```python
from build123d import *

# Parameters (mm, degrees)
EXTRUDE_1_DEPTH = 1
SKETCH_3_R      = 1.5
SKETCH_3_R_2    = 2.75
EXTRUDE_2_DEPTH = 6
EXTRUDE_3_DEPTH = 3


with BuildPart() as part:
    # 草图1 → 凸台-拉伸1 (new body)
    with BuildSketch(Plane.XY):
        with BuildLine():
            Line((-15.782608696, 8.75), (17.217391304, 8.75))
            ThreePointArc((17.217391304, 8.75), (20.045818429, 7.578427125), (21.217391304, 4.75))
            Line((21.217391304, 4.75), (21.217391304, -3.25))
            ThreePointArc((21.217391304, -3.25), (20.045818429, -6.078427125), (17.217391304, -7.25))
            Line((17.217391304, -7.25), (-15.782608696, -7.25))
            ThreePointArc((-15.782608696, -7.25), (-18.61103582, -6.078427125), (-19.782608696, -3.25))
            Line((-19.782608696, -3.25), (-19.782608696, 4.75))
            ThreePointArc((-19.782608696, 4.75), (-18.61103582, 7.578427125), (-15.782608696, 8.75))
        make_face()
    extrude(amount=EXTRUDE_1_DEPTH)

    # 草图3 → 凸台-拉伸2 (add)
    with BuildSketch(Plane.XY.offset(1)):
        with Locations((2.717391304, 5.25)):
            Circle(SKETCH_3_R)
        with Locations((9.717391304, 5.25)):
            Circle(SKETCH_3_R)
        with Locations((6.217391304, -2.75)):
            Circle(SKETCH_3_R_2)
        with Locations((15.717391304, -0.75)):
            Circle(SKETCH_3_R_2)
    extrude(amount=EXTRUDE_2_DEPTH)

    # 草图4 → 凸台-拉伸3 (add)
    with BuildSketch(Plane.XY):
        Polygon((-8.282608696, 2.75), (-8.282608696, 6.75), (-12.282608696, 6.75), (-12.282608696, 2.75), (-16.282608696, 2.75), (-16.282608696, -1.25), (-12.282608696, -1.25), (-12.282608696, -5.25), (-8.282608696, -5.25), (-8.282608696, -1.25), (-4.282608696, -1.25), (-4.282608696, 2.75), align=None)
    extrude(amount=EXTRUDE_3_DEPTH)


solid = part.part
```
Here's how the part is built. I have some questions about the finished solid (model axes, mm). A direction names the side the tool comes from. Give positions to 0.01 mm unless a question says otherwise; leave off trailing zeros. Loops run counter-clockwise (first coordinate to the right, second up) from the corner with the lowest first, then second, coordinate; pieces in that order, holes last. Notation, with made-up numbers: M 13,86 L 21,86 A19 cw 21,93 Z; hole C 75.25,45 d9. An arc over 180 degrees is marked long. Use one line per item in the form item = value. Start each with the question number.
Q1. Thinking about a two-plate mould opening in X: for faces 5 (the cylindrical face through (5.621, -5.435, 3.958)), 6 (the flat face through (6, -3, 7)), 7 (the cylindrical face through (-18.58, -6.11, 0.49)), which applies, +X half, -X half, draft (parallel to the pull), parting line (faces both ways), or undercut?
Q2. If we section it at C-C (x = -9): Write out the boundary of the cut face in (y, z), then the cut area to 3 significant figures.
Q3. Which directions (+Z, -Z, +X, -X, +Y, -Y) give clear straight access to the entire face, cutting with the end or side of a thin tool? Please do faces 1 (the flat face through (-8.283, 5, 2)), 2 (the cylindrical face through (8.22, 5.32, 3.96)), 3 (the flat face through (-14, -1.25, 2)), 4 (the flat face through (-6, -1.25, 2)).
Q4. I need wall thicknesses on line 1 along Z through (x, y) = (6.5, 1.5); line 2 along X through (y, z) = (4.5, 2.5); line 3 along Y through (x, z) = (4, 6.75). Which ranges of each line are inside material? Lowest first, please.
Q5. Will these pins go through, and if not, where does the flat tip stop? pin 1 Ø1 at (y, z) = (4, 2) entering from +X; pin 2 Ø1 at (x, z) = (-6.5, 2) entering from +Y; pin 3 Ø1 at (y, z) = (0, 2) entering from -X; pin 4 Ø1 at (x, z) = (-1, 3.5) entering from -Y.
Q6. If we section it at A-A (z = 2.25): Write out the boundary of the cut face in (x, y).
Q7. If we section it at D-D (z = 5): Write out the boundary of the cut face in (x, y), then the cut area to 3 significant figures.
Q8. If we section it at B-B (y = -1.75): Write out the boundary of the cut face in (x, z).
Taken from the geometry:
q1.face_5 = undercut
q1.face_6 = draft
q1.face_7 = -X half
q2.outline = M -7.25,0 L 8.75,0 L 8.75,1 L 6.75,1 L 6.75,3 L -5.25,3 L -5.25,1 L -7.25,1 Z
q2.area = 40.0 mm^2
q3.face_1 = +Z, +Y
q3.face_2 = +Z
q3.face_3 = +Z, -X, -Y
q3.face_4 = +Z, -Y
q4.line_1 = 0 to 1
q4.line_2 = -12.28 to -8.28, 1.42 to 4.02, 8.42 to 11.02
q4.line_3 = -4.38 to -1.12, 4.47 to 6.03
q5.pin_1 = 11.02
q5.pin_2 = 2.75
q5.pin_3 = -16.28
q5.pin_4 = through
q6.outline = M -16.28,-1.25 L -12.28,-1.25 L -12.28,-5.25 L -8.28,-5.25 L -8.28,-1.25 L -4.28,-1.25 L -4.28,2.75 L -8.28,2.75 L -8.28,6.75 L -12.28,6.75 L -12.28,2.75 L -16.28,2.75 Z; C 2.72,5.25 d3; C 6.22,-2.75 d5.5; C 9.72,5.25 d3; C 15.72,-0.75 d5.5
q7.outline = C 2.72,5.25 d3; C 6.22,-2.75 d5.5; C 9.72,5.25 d3; C 15.72,-0.75 d5.5
q7.area = 61.7 mm^2
q8.outline = M -19.78,0 L 21.22,0 L 21.22,1 L 18.28,1 L 18.28,7 L 13.16,7 L 13.16,1 L 8.78,1 L 8.78,7 L 3.66,7 L 3.66,1 L -8.28,1 L -8.28,3 L -12.28,3 L -12.28,1 L -19.78,1 Z
